Autodesk Inventor part; units mm, degrees
ref_plane "作業平面3" through (0, -75, 0) normal (0, 0.7071, 0.7071) x (-1, 0, 0)
ref_plane "YZ Plane" through (0, 0, 0) normal (1, 0, 0) x (0, 1, 0)
ref_plane "XZ Plane" through (0, 0, 0) normal (0, 1, 0) x (-1, 0, 0)
ref_plane "作業平面1" through (0, 0, 0) normal (0, 0, 1) x (1, 0, 0)
sketch "スケッチ2" plane through (0, 0, 0) normal (0, 0, 1) x (1, 0, 0)
  line L0 (120, -56.75) -> (-20, -56.75)
  line L1 (-20, -56.75) -> (-20, -93.25)
  line L2 (-20, -93.25) -> (120, -93.25)
  line L3 (120, -93.25) -> (120, -56.75)
  circle A0 centre (0, -75) radius 6 construction
  circle A1 centre (0, -75) radius 75 construction
  point P0 (0, 0)
  dimension "d1" = 150
  dimension "d2" = 18.25
  dimension "d3" = 18.25
  dimension "d4" = 20
  dimension "d29" = 120
extrude "押し出し1" add sketch "スケッチ2" along normal blind 6
sketch "スケッチ3" plane through (0, 0, 6) normal (0, 0, 1) x (1, 0, 0)
  circle A0 centre (0, -75) radius 6 construction
  circle A1 centre (0, -75) radius 6.25
  line L0 (0, -68.75) -> (-38.1, -68.75) construction
  line L1 (-38.1, -68.75) -> (-38.1, -81.25) construction
  line L2 (-38.1, -81.25) -> (0, -81.25) construction
  line L3 (0, -81.25) -> (0, -68.75) construction
  line L4 (-20, -68) -> (-20, -81.25)
  line L5 (0, -82) -> (0, -68.75)
  line L6 (-20, -56.75) -> (-20, -93.25)
  line L7 (-20, -69.25) -> (2.4495, -69.25)
  line L8 (2.4495, -69.25) -> (2.4495, -80.75)
  line L9 (2.4495, -80.75) -> (-20, -80.75)
  line L10 (-20, -80.75) -> (-20, -69.25)
  point P0 (0, 0)
  point P1 (-2.4495, -80.75)
  point P2 (-2.4495, -69.25)
  point P3 (0, -80.75)
  point P4 (0, -69.25)
  point P5 (0, -81.25)
  dimension "d8" = 12.5
  dimension "d30" = 11.5
extrude "押し出し2" cut sketch "スケッチ3" against normal blind 12.5 contours A1 L8 | L8 L9 L5 L7 | L5 L9 A1 L7 | A1 L9 L4 L7
fillet "フィレット1" radius 10 2 edges at (-20, -80.75, 3) (-20, -69.25, 3)
ref_plane "作業平面2" through (-20, -75, 0) normal (0, -1, 0) x (1, 0, 0)
sketch "スケッチ4" plane through (0, 0, 6) normal (0, 0, 1) x (1, 0, 0)
  line L0 (-20, -93.25) -> (120, -93.25)
  line L1 (120, -56.75) -> (-20, -56.75)
  line L2 (120, -93.25) -> (120, -56.75)
  point P0 (0, 0)
  point P1 (105, -75)
  dimension "d25" = 15
  dimension "d26" = 36.5
  dimension "d27" = 18.25
hole "穴1" at (105, -75, 6) direction (0, 0, -1) diameter 6.6 end through all
ref_plane "作業平面3" through (0, -75, 0) normal (0, 0.7071, 0.7071) x (-1, 0, 0)
sketch "スケッチ5" plane through (0, 0, 0) normal (0, 0, 1) x (1, 0, 0)
  circle A0 centre (105, -75) radius 3.3 construction
  arc A1 (-20, -59.25) -> (-10, -69.25) centre (-10, -59.25) ccw construction
  line L0 (-10, -69.25) -> (2.4495, -69.25) construction
  arc A2 (2.4495, -80.75) -> (2.4495, -69.25) centre (0, -75) ccw construction
  line L1 (2.4495, -80.75) -> (-10, -80.75) construction
  arc A3 (-10, -80.75) -> (-20, -90.75) centre (-10, -90.75) ccw construction
  line L2 (-20, -90.75) -> (-20, -93.25) construction
  line L3 (-20, -93.25) -> (120, -93.25) construction
  line L4 (120, -93.25) -> (120, -56.75) construction
  line L5 (120, -56.75) -> (-20, -56.75) construction
  line L6 (-20, -56.75) -> (-20, -59.25) construction
  line L7 (123, -56.75) -> (87, -56.75)
  line L8 (87, -56.75) -> (87, -93.25)
  line L9 (87, -93.25) -> (123, -93.25)
  line L10 (123, -93.25) -> (123, -56.75)
  line L11 (120, -93.25) -> (120, -56.75)
  line L12 (90, -90.25) -> (120, -90.25)
  line L13 (120, -90.25) -> (120, -59.75)
  line L14 (120, -59.75) -> (90, -59.75)
  line L15 (90, -59.75) -> (90, -90.25)
  line L16 (90, -90.25) -> (120, -59.75) construction
  line L17 (120, -90.25) -> (90, -59.75) construction
  line L18 (87, -85.25) -> (123, -85.25)
  line L19 (123, -85.25) -> (123, -64.75)
  line L20 (123, -64.75) -> (87, -64.75)
  line L21 (87, -64.75) -> (87, -85.25)
  circle A4 centre (105, -75) radius 3.3
  line L22 (87, -85.25) -> (123, -64.75) construction
  line L23 (123, -85.25) -> (87, -64.75) construction
  line L24 (95, -93.25) -> (115, -93.25)
  line L25 (115, -93.25) -> (115, -56.75)
  line L26 (115, -56.75) -> (95, -56.75)
  line L27 (95, -56.75) -> (95, -93.25)
  line L28 (95, -93.25) -> (115, -56.75) construction
  line L29 (115, -93.25) -> (95, -56.75) construction
  point P0 (0, 0)
  point P1 (95, -93.25)
  point P2 (95, -90.25)
  point P3 (90, -85.25)
  point P4 (95, -59.75)
  point P5 (90, -64.75)
  point P6 (120, -85.25)
  point P7 (115, -90.25)
  point P8 (115, -93.25)
  point P9 (115, -59.75)
  point P10 (120, -64.75)
  dimension "d31" = 3
  dimension "d34" = 30.5
  dimension "d35" = 3
  dimension "d36" = 3
  dimension "d37" = 3
  dimension "d38" = 8
  dimension "d39" = 8
extrude "押し出し3" add sketch "スケッチ5" against normal blind 4 contours L10 L20 L11 L7 | L11 L14 L25 L7 | L10 L9 L11 L18 | L27 L14 L15 L20 L8 L7 | L9 L25 L12 L11 | L18 L15 L12 L27 L9 L8
sketch "スケッチ6" plane through (120, -93.25, 0) normal (1, 0, 0) x (0, 0, -1)
  line L0 (0, 8) -> (0, 28.5)
  line L1 (0, 36.5) -> (-6, 36.5)
  line L2 (-6, 0) -> (-6, 36.5)
  line L3 (0, 0) -> (-6, 0)
  line L4 (0, 0) -> (0, 3)
  line L5 (0, 3) -> (0, 8)
  line L6 (0, 28.5) -> (0, 33.5)
  line L7 (0, 33.5) -> (0, 36.5)
  point P0 (0, 93.25)
extrude "押し出し4" add sketch "スケッチ6" along normal up to surface (3 mm away)
fillet "フィレット2" radius 2 8 edges at (-20, -56.75, 3) (-20, -93.25, 3) (87, -56.75, -2) (87, -93.25, -2) (87, -64.75, -2) (87, -85.25, -2) (123, -64.75, -2) (123, -85.25, -2)
fillet "フィレット2" radius 0.5 16 edges at (115, -59.75, -2) (120, -64.75, -2) (120, -85.25, -2) (115, -90.25, -2) (95, -59.75, -2) (90, -64.75, -2) (90, -62.25, -4) (92.5, -59.75, -4) (117.5, -59.75, -4) (120, -62.25, -4) (120, -87.75, -4) (117.5, -90.25, -4) (95, -90.25, -2) (90, -85.25, -2) (90, -87.75, -4) (92.5, -90.25, -4)
sketch "スケッチ7" plane through (20.6125, 13, 6) normal (0, 0, 1) x (1, 0, 0)
  arc A0 (3.9922, -80.75) -> (-0.2106, -72.4528) centre (-20.6125, -88) ccw
  circle A1 centre (-20.6125, -88) radius 31.5 construction
  circle A2 centre (7.9653, -101.25) radius 2.75 construction
  line L0 (-18, -106.25) -> (105, -106.25) construction
  arc A3 (-18.163, -93.75) -> (-18.163, -82.25) centre (-20.6125, -88) ccw
  line L1 (-38.6125, -106.25) -> (100.3875, -106.25)
  point P0 (0, 0)
  dimension "d48" = 63
  dimension "d46" = 5.5
  dimension "d47" = 5
hole "穴2" at (28.5777, -88.25, 6) direction (0, 0, -1) diameter 5.5 end through all
sketch "スケッチ8" plane through (0, 0, 6) normal (0, 0, 1) x (1, 0, 0)
  circle A0 centre (28.5777, -88.25) radius 2.75 construction
  arc A1 (121, -93.25) -> (123, -91.25) centre (121, -91.25) ccw construction
  line L0 (123, -91.25) -> (123, -58.75) construction
  arc A2 (123, -58.75) -> (121, -56.75) centre (121, -58.75) ccw construction
  line L1 (-18, -56.75) -> (121, -56.75) construction
  arc A3 (-18, -56.75) -> (-20, -58.75) centre (-18, -58.75) ccw construction
  line L2 (-20, -58.75) -> (-20, -59.25) construction
  arc A4 (-20, -59.25) -> (-10, -69.25) centre (-10, -59.25) ccw construction
  line L3 (-10, -69.25) -> (2.4495, -69.25) construction
  arc A5 (2.4495, -80.75) -> (2.4495, -69.25) centre (0, -75) ccw construction
  line L4 (2.4495, -80.75) -> (-10, -80.75) construction
  arc A6 (-10, -80.75) -> (-20, -90.75) centre (-10, -90.75) ccw construction
  line L5 (-20, -90.75) -> (-20, -91.25) construction
  arc A7 (-20, -91.25) -> (-18, -93.25) centre (-18, -91.25) ccw construction
  line L6 (-18, -93.25) -> (121, -93.25) construction
  circle A8 centre (105, -75) radius 3.3 construction
  line L7 (23.5777, -91) -> (33.5777, -91)
  line L8 (33.5777, -91) -> (33.5777, -85.5) construction
  line L9 (33.5777, -85.5) -> (23.5777, -85.5)
  line L10 (23.5777, -85.5) -> (23.5777, -91) construction
  circle A9 centre (28.5777, -88.25) radius 2.75
  line L11 (23.5777, -91) -> (33.5777, -85.5) construction
  line L12 (33.5777, -91) -> (23.5777, -85.5) construction
  arc A10 (33.5777, -91) -> (33.5777, -85.5) centre (33.5777, -88.25) ccw
  arc A11 (23.5777, -85.5) -> (23.5777, -91) centre (23.5777, -88.25) ccw
  point P0 (0, 0)
  dimension "d55" = 10
extrude "押し出し5" cut sketch "スケッチ8" against normal through all
equation "\"d3\" = d2"
equation "\"d9\" = d8"
equation "\"d35\" = d31"
equation "\"d36\" = d31"
equation "\"d37\" = d31"
equation "\"d39\" = d38"
properties part number "wheel_mount._brake_01ipt" material "アルミニウム 6061"
Can you work these out from the model? Positions are in its coordinate system, mm. A direction names the side the tool comes from. Round coordinates to 2 decimals unless told otherwise and drop trailing zeros. Order: outer loops, then holes, each group sorted by start corner. A loop starts at its lowest first (then second) coordinate and runs counter-clockwise, first axis right, second up.
(1) If I drill on L1, parallel to X at y = -63, z = -2.25; L2, parallel to Y at x = 105, z = 3.5; L3, parallel to X at y = -75, z = 1.75, over which ranges is the centre line in solid material (lowest first)?
Results are:
L1: x = 87.02 to 90, 120 to 122.98
L2: y = -93.25 to -78.3, -71.7 to -56.75
L3: x = 6.25 to 101.7, 108.3 to 123
(2) If we section it at D-D (x = 14): Please give me the cut outline in (y, z), plus the area to 3 significant figures.
Results are:
outline: (-93.25, 0) - (-56.75, 0) - (-56.75, 6) - (-93.25, 6) - close
area: 219 mm2
(3) If we section it at A-A (x = 105): Please give me the cut outline in (y, z), plus the area to 3 significant figures.
Results are:
outline: (-93.25, 0) - (-78.3, 0) - (-78.3, 6) - (-93.25, 6) - close; (-71.7, 0) - (-56.75, 0) - (-56.75, 6) - (-71.7, 6) - close
area: 179 mm2
(4) On a 3-axis mill with a long thin cutter (end or side, diameter ignored), from which of +Z, -Z, +X, -X, +Y, -Y can I reach the whole of each face in a straight line? I mean faces 1 (the face through (95, -58, -2)), 2 (the face through (20.83, -88.19, 3.04)), 3 (the face through (87, -61, -2)). Say none if no direction works.
Results are:
face 1: -Z, +Y, -Y
face 2: +Z, -Z
face 3: -Z, -X, +Y, -Y
(5) If we section it at C-C (z = 3.5): Please give me the cut outline in (x, y).
Results are:
outline: (-20, -91.25) arc R2 ccw to (-18, -93.25) - (123, -93.25) - (123, -56.75) - (-18, -56.75) arc R2 ccw to (-20, -58.75) - (-20, -59.25) arc R10 ccw to (-10, -69.25) - (2.45, -69.25) arc R6.25 cw to (2.45, -80.75) - (-10, -80.75) arc R10 ccw to (-20, -90.75) - close; hole (23.58, -91) - (33.58, -91) arc R2.75 ccw to (33.58, -85.5) - (23.58, -85.5) arc R2.75 ccw to start; hole circle Ø6.6 at (105, -75)
(6) If we section it at B-B (y = -75): Please give me the cut outline in (x, z).
Results are:
outline: (6.25, 0) - (101.7, 0) - (101.7, 6) - (6.25, 6) - close; (108.3, 0) - (123, 0) - (123, 6) - (108.3, 6) - close
(7) We'd pull the mould along X, two halves only. Please class faces 4 (the face through (120, -91, -4)), 5 (the face through (95, -92, -2)), 6 (the face through (6.25, -75.1, 3.04)): +X half, -X half, draft (parallel to the pull), parting line (faces both ways), or undercut.
Results are:
face 4: draft
face 5: undercut
face 6: -X half
(8) I'm going to push flat-ended pins straight in: pin 1 (5 mm diameter, centred on y = -88, z = 1, fed in from -X); pin 2 (3 mm diameter, centred on y = -92, z = -3, fed in from -X); pin 3 (2 mm diameter, centred on y = -74, z = -1.5, fed in from -X); pin 4 (2 mm diameter, centred on x = 69.5, y = -84, fed in from -Z). Where does each tip first touch, or does it pass through?
Results are:
pin 1: stops at x = -20
pin 2: stops at x = 87
pin 3: passes through
pin 4: stops at z = 0
